from build123d import *

# Parameters (mm, degrees)
F0_R     = 3.5
F0_R_2   = 2.25
F1_DEPTH = 2
F2_DEPTH = 5
F3_R     = 1.99999


# Not quite as in the source:
# - a fillet or chamfer is up to 0.001 mm smaller than in the source, because OpenCascade refuses the exact size


with BuildPart() as f1:
    # F0 (on Top) → F1 (new body)
    with BuildSketch(Plane.XY):
        Circle(F0_R)
        Circle(F0_R_2, mode=Mode.SUBTRACT)
        Circle(F0_R_2)
    extrude(amount=-F1_DEPTH)

    # F0 (on Top) → F2 (join)
    with BuildSketch(Plane.XY):
        Circle(F0_R_2)
    extrude(amount=F2_DEPTH)

    # F3 (radius 2 in the source; OpenCascade refuses exactly that, so slightly less here)
    f3_edges = [f1.edges().sort_by_distance(p)[0] for p in [
        (-2.25, 0, 5),
        (-3.5, 0, -2),
    ]]
    fillet(f3_edges, radius=F3_R)


solid = f1.part
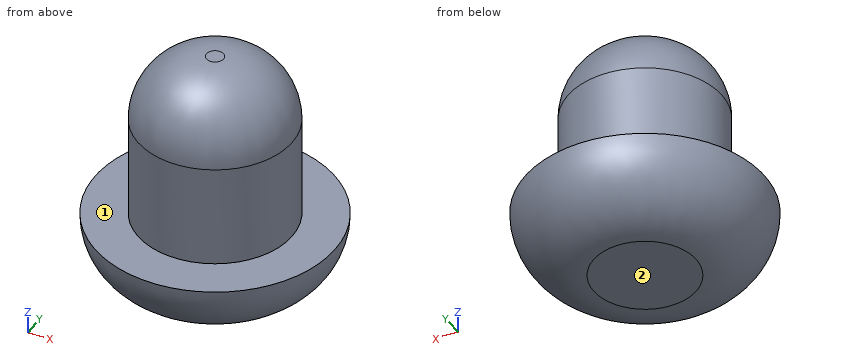
Source: CAD feature listing. Evaluate the final solid. Frame: model axes, mm. Face numbers are marked on the shaded views. A direction names the side the tool comes from. Round coordinates to 2 decimals unless told otherwise and drop trailing zeros. Loops run counter-clockwise (first coordinate to the right, second up) from the corner with the lowest first, then second, coordinate; pieces in that order, holes last.
Q1. Section A-A, the plane z = 2.75. Return loops of the section in (x, y), plus the area to 3 significant figures.
Q2. First-contact query: P1, Ø1, axis at x = 1.5, z = 2.5, coming from the -Y side. Flat tip, straight axial feed; report the tip coordinate or a pass-through.
Q3. Ray query, line 1 (Y direction, x = 0, z = 1.5); line 2 (X direction, y = 1.25, z = 0.5); line 3 (Z direction, x = 1, y = 2.5). Return the intervals inside material, ascending.
Q4. Access query for the marked faces 1 and 2. Directions: +Z, -Z, +X, -X, +Y, -Y. A direction counts if a zero-diameter tool reaches every point of the face in a straight line with its end or side. Return the directions, or none.
Solutions:
1. outline: circle Ø4.5 at (0, 0)
1. area: 15.9 mm2
2. P1: stops at y = -2.02
3. line 1: y = -2.25 to 2.25
3. line 2: x = -1.87 to 1.87
3. line 3: z = -1.61 to 0
4. face 1: +Z
4. face 2: -Z, +X, -X, +Y, -Y
